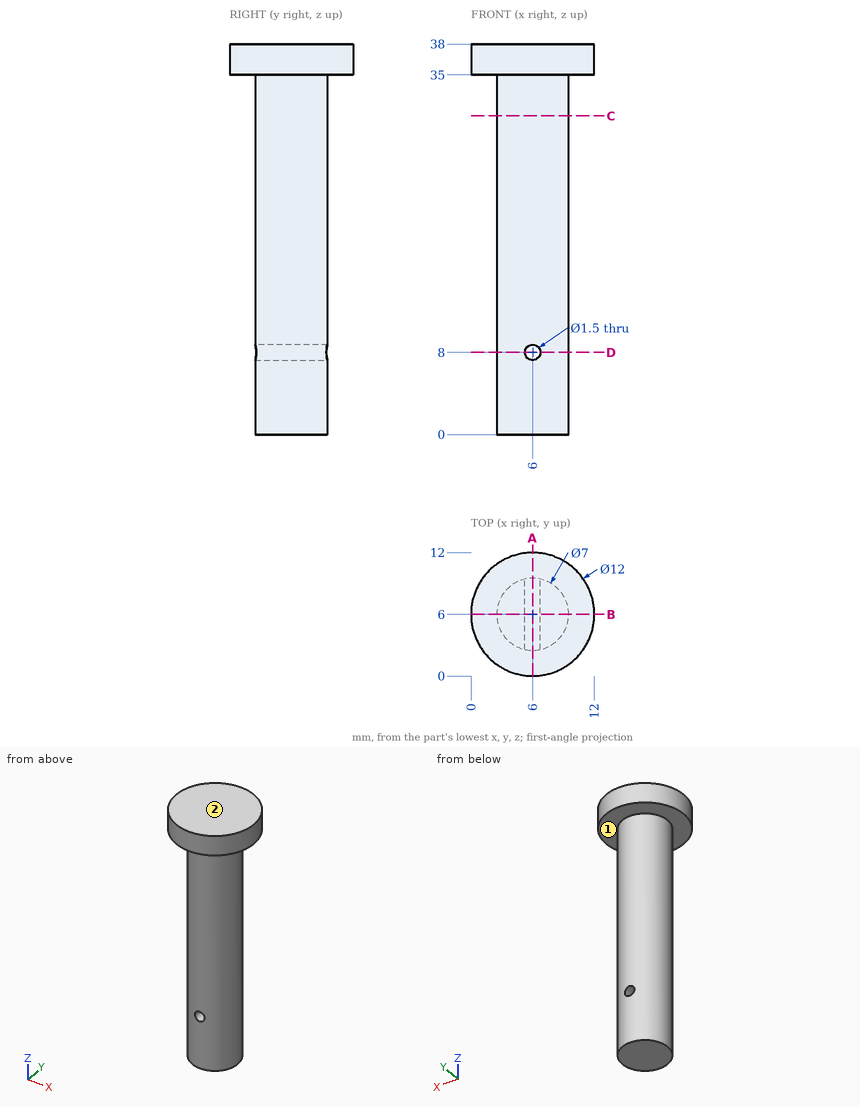
Here's the drawing with two shaded views (mm, measured from the low corner). I have some questions. A direction names the side the tool comes from. Coordinates: 2 decimals unless noted, no trailing zeros. Loops run counter-clockwise (first coordinate to the right, second up) from the corner with the lowest first, then second, coordinate; pieces in that order, holes last. Notation, with made-up numbers: M 40.25,88 L 91.25,88 A23 cw 91.25,109 Z; hole C 20.25,73 d8. An arc over 180 degrees is marked long. Put each result on its own line as item: value. Start each with the question number.
(1) Imagine slicing it at B-B on y = 6. List the corners of the cut face in (x, z) for me, and give its area (3 significant figures).
(2) Which directions (+Z, -Z, +X, -X, +Y, -Y) give clear straight access to the entire face, cutting with the end or side of a thin tool? Please do the marked faces 1 and 2.
(3) Will these pins go through, and if not, where does the flat tip stop? pin 1 Ø4 at (y, z) = (9, 12) entering from -X; pin 2 Ø5 at (y, z) = (6.5, 19) entering from +X; pin 3 Ø4 at (x, z) = (5, 17) entering from -Y.
(4) Imagine slicing it at C-C on z = 31. List the corners of the cut face in (x, y) for me.
(5) Imagine slicing it at A-A on x = 6. List the corners of the cut face in (y, z) for me.
(6) Imagine slicing it at D-D on z = 8. List the corners of the cut face in (x, y) for me.
(7) I need wall thicknesses on probe 1 along Z at (x, y) = (6, 7); probe 2 along X at (y, z) = (5.5, 8); probe 3 along Y at (x, z) = (5.75, 26). Which ranges of each line are inside material? Lowest first, please.
Worked answers:
1. outline: M 0,35 L 2.5,35 L 2.5,0 L 9.5,0 L 9.5,35 L 12,35 L 12,38 L 0,38 Z; hole C 6,8 d1.5
1. area: 279 mm2
2. face 1: -Z
2. face 2: +Z, +X, -X, +Y, -Y
3. pin 1: stops at x = 2.65
3. pin 2: stops at x = 9.5
3. pin 3: stops at y = 2.5
4. outline: C 6,6 d7
5. outline: M 0,35 L 2.5,35 L 2.5,8.75 L 9.5,8.75 L 9.5,35 L 12,35 L 12,38 L 0,38 Z; M 2.5,0 L 9.5,0 L 9.5,7.25 L 2.5,7.25 Z
6. outline: M 5.25,2.58 L 5.25,9.42 A3.5 ccw Z; M 6.75,2.58 A3.5 ccw 6.75,9.42 Z
7. probe 1: z = 0 to 7.25, 8.75 to 38
7. probe 2: x = 2.54 to 5.25, 6.75 to 9.46
7. probe 3: y = 2.51 to 9.49
